Could you check a few things on this model? Use its own coordinates, in mm. A direction names the side the tool comes from. Coordinates: 2 decimals unless noted, no trailing zeros. Order: outer loops, then holes, each group sorted by start corner. A loop starts at its lowest first (then second) coordinate and runs counter-clockwise, first axis right, second up. Notation, with made-up numbers: M 27,6.25 L 45,6.25 A14 ccw 45,21.25 Z; hole C 34,-14.75 d4. An arc over 180 degrees is marked long. Put each result on its own line as item: value. Start each with the question number.
```python
from build123d import *

# Parameters (mm, degrees)
SKETCH_2_W      = 390
SKETCH_2_H      = 390
SKETCH_2_R      = 1.5
SKETCH_2_W_2    = 230
SKETCH_2_H_2    = 149
SKETCH_2_W_3    = 160
SKETCH_2_H_3    = 150
EXTRUDE_1_DEPTH = 6


with BuildPart() as part:
    # 草图2 → 凸台-拉伸1 (new body)
    with BuildSketch(Plane(origin=(0, 0, 0), x_dir=(1, 0, 0), z_dir=(0, 1, 0))):
        Rectangle(SKETCH_2_W, SKETCH_2_H)
        with Locations(Location((185, -185, 0), (0, 0, 270))):
            Circle(SKETCH_2_R, mode=Mode.SUBTRACT)
        with Locations(Location((-185, 185, 0), (0, 0, 270))):
            Circle(SKETCH_2_R, mode=Mode.SUBTRACT)
        with Locations(Location((110, 21.5, 0), (0, 0, 270))):
            Circle(SKETCH_2_R, mode=Mode.SUBTRACT)
        with Locations(Location((-110, 178.5, 0), (0, 0, 270))):
            Circle(SKETCH_2_R, mode=Mode.SUBTRACT)
        with Locations(Location((-110, 21.5, 0), (0, 0, 270))):
            Circle(SKETCH_2_R, mode=Mode.SUBTRACT)
        with Locations(Location((110, 178.5, 0), (0, 0, 270))):
            Circle(SKETCH_2_R, mode=Mode.SUBTRACT)
        with Locations(Location((-185, -185, 0), (0, 0, 270))):
            Circle(SKETCH_2_R, mode=Mode.SUBTRACT)
        with Locations(Location((185, 185, 0), (0, 0, 270))):
            Circle(SKETCH_2_R, mode=Mode.SUBTRACT)
        with Locations((0, 100)):
            Rectangle(SKETCH_2_W_2, SKETCH_2_H_2, mode=Mode.SUBTRACT)
        with Locations((0, -89.5)):
            Rectangle(SKETCH_2_W_3, SKETCH_2_H_3, mode=Mode.SUBTRACT)
        Polygon((-135, -70), (-105, -90), (-135, -30), (-165, -90), align=None, mode=Mode.SUBTRACT)
        Polygon((135, -70), (165, -90), (135, -30), (105, -90), align=None, mode=Mode.SUBTRACT)
    extrude(amount=EXTRUDE_1_DEPTH)


solid = part.part
```
Item 1: If we mould it in two halves opening along X, with no side actions, what happens to faces 1 (the flat face through (150, 3, 60)), 2 (the flat face through (-3, 6, -3)), 3 (the flat face through (-150, 3, 60))? For each: released by +X, released by -X, zero draft, split by the parting line, or undercut.
Item 2: I need wall thicknesses on probe 1 along Z at (x, y) = (-185, 3.3); probe 2 along Z at (x, y) = (68, 0.5). Which ranges of each line are inside material? Lowest first, please.
Item 3: For faces 4 (the flat face through (-3, 0, -3)), 5 (the flat face through (-120, 3, 60)), which set-ups out of +Z, -Z, +X, -X, +Y, -Y let a thin tool reach every point of the face, with its end or its side?
Item 4: If we section it at D-D on y = 4.5: State how many separate pieces and enclosed holes the cut face has, then the cut area to 3 significant figures.
Item 5: For pin 1 Ø2.5 at (x, z) = (185, 185) entering from -Y, with a flat end and sliding along its axis, tell me the tip position at first contact or that it passes through.
Item 6: If we section it at B-B on z = 23: Write out the boundary of the cut face in (x, y), then the cut area to 3 significant figures.
Item 7: If we section it at A-A on z = 74.5: Write out the boundary of the cut face in (x, y), then the cut area to 3 significant figures.
Item 8: If we section it at C-C on x = 59.5: Write out the boundary of the cut face in (y, z), then the cut area to 3 significant figures.
Geometry check:
1. face 1: undercut
1. face 2: zero draft
1. face 3: undercut
2. probe 1: z = -195 to -186.5, -183.5 to 183.5, 186.5 to 195
2. probe 2: z = -195 to -174.5, -25.5 to 14.5, 164.5 to 195
3. face 4: +Z, -Z, +X, -X, -Y
3. face 5: +Y, -Y
4. separate pieces: 1
4. enclosed holes: 12
4. area: 91,400 mm²
5. pin 1: passes through
6. outline: M -195,0 L -80,0 L -80,6 L -195,6 Z; M 80,0 L 195,0 L 195,6 L 80,6 Z
6. area: 1,380 mm²
7. outline: M -195,0 L -157.25,0 L -157.25,6 L -195,6 Z; M -141.75,0 L -128.25,0 L -128.25,6 L -141.75,6 Z; M -112.75,0 L -80,0 L -80,6 L -112.75,6 Z; M 80,0 L 112.75,0 L 112.75,6 L 80,6 Z; M 128.25,0 L 141.75,0 L 141.75,6 L 128.25,6 Z; M 157.25,0 L 195,0 L 195,6 L 157.25,6 Z
7. area: 1,010 mm²
8. outline: M 0,-195 L 6,-195 L 6,-174.5 L 0,-174.5 Z; M 0,-25.5 L 6,-25.5 L 6,14.5 L 0,14.5 Z; M 0,164.5 L 6,164.5 L 6,195 L 0,195 Z
8. area: 546 mm²
